from build123d import *

# Parameters (mm, degrees)
EXTRUDE_1_DEPTH         = 5
HOLE_WIZARD_A_0_234_3_D = 3.1999936
PATTERN_LINEAR_1_COUNT  = 3
PATTERN_LINEAR_1_PITCH  = 8
HOLE_WIZARD_A_0_234_4_D = 4


with BuildPart() as part:
    # Эскиз1 → Бобышка-Вытянуть1 (new body)
    with BuildSketch(Plane.XZ):
        with BuildLine():
            Line((-6, 31.613261479), (-6, 0))
            Line((-6, 0), (6, 0))
            Line((6, 0), (6, 37.436574312))
            ThreePointArc((6, 37.436574312), (6.281622528, 39.793084297), (7.110627862, 42.016865021))
            Line((7.110627862, 42.016865021), (12.856242572, 53.167883716))
            ThreePointArc((12.856242572, 53.167883716), (11.13261, 58.555748855), (5.744744861, 56.832116284))
            Line((5.744744861, 56.832116284), (-4.889372139, 36.193552189))
            ThreePointArc((-4.889372139, 36.193552189), (-5.718377472, 33.969771464), (-6, 31.613261479))
        make_face()
    extrude(amount=-EXTRUDE_1_DEPTH)

    # Диаметр отверстия A (0.234)3 (through all)
    with Locations(Plane(origin=(0, 0, 4), x_dir=(0, 0, -1), z_dir=(0, -1, 0))):
        with Locations((0, 0)):
            hole_wizard_a_0_234_3 = Hole(HOLE_WIZARD_A_0_234_3_D / 2)

    # Линейный массив1: Диаметр отверстия A (0.234)3 ×3
    with Locations(*[(0, 0, i * PATTERN_LINEAR_1_PITCH) for i in range(1, PATTERN_LINEAR_1_COUNT)]):
        add(hole_wizard_a_0_234_3, mode=Mode.SUBTRACT)

    # Диаметр отверстия A (0.234)4 (through all)
    with Locations(Plane(origin=(9.3, 0, 55), x_dir=(0, 0, -1), z_dir=(0, -1, 0))):
        with Locations((0, 0), (15.76854256, -8.11912081)):
            Hole(HOLE_WIZARD_A_0_234_4_D / 2)


solid = part.part
Source: CAD feature listing. Evaluate the final solid. Frame: model axes, mm. Coordinates: 2 decimals unless noted, no trailing zeros. Loops run counter-clockwise (first coordinate to the right, second up) from the corner with the lowest first, then second, coordinate; pieces in that order, holes last. Notation, with made-up numbers: (-6.5, 10) -> (52.5, 10) arc R23 ccw to (52.5, 18) -> close; hole circle Ø9 at (68.25, -6.5). An arc over 180 degrees is marked (long way). Answer in a Markdown table with one row per item. Add a question column.
Q1. Section B-B on z = 4. Return the cut outline in (x, y), and give its area (3 significant figures).
Q2. Section C-C on x = 0. Return the cut outline in (y, z), and give its area (3 significant figures).
Q3. Ray query, line 1 along X through (y, z) = (2.2, 4); line 2 along X through (y, z) = (0.3, 6); line 3 along X through (y, z) = (4.6, 55). Return the intervals inside material, ascending.
Q4. Section A-A on x = 10.5. Return the cut outline in (y, z), and give its area (3 significant figures).
Q5. Section D-D on y = 2.05. Return the cut outline in (x, z), and give its area (3 significant figures).
Q6. Pull-direction query (X, two-part tool) for faces 1 (the face through (0, 2, 0)), 2 (the face through (6, 2, 18)), 3 (the face through (0.481, 2.535, 13.526)), 4 (the face through (-6, 2, 16)); classes: pulls with the +X half, pulls with the -X half, needs draft (parallel to the pull), parting line crosses it, or undercut.
Computed values:
| question | item | result |
|---|---|---|
| 1 | outline | (-6, 0) -> (-1.6, 0) -> (-1.6, 5) -> (-6, 5) -> close; (1.6, 0) -> (6, 0) -> (6, 5) -> (1.6, 5) -> close |
| 1 | area | 44.0 mm^2 |
| 2 | outline | (0, 0) -> (5, 0) -> (5, 2.4) -> (0, 2.4) -> close; (0, 5.6) -> (5, 5.6) -> (5, 10.4) -> (0, 10.4) -> close; (0, 13.6) -> (5, 13.6) -> (5, 18.4) -> (0, 18.4) -> close; (0, 21.6) -> (5, 21.6) -> (5, 37.62) -> (0, 37.62) -> close; (0, 40.85) -> (5, 40.85) -> (5, 45.68) -> (0, 45.68) -> close |
| 2 | area | 164 mm^2 |
| 3 | line 1 | x = -6 to -1.6, 1.6 to 6 |
| 3 | line 2 | x = -6 to 6 |
| 3 | line 3 | x = 4.8 to 7.3, 11.3 to 13.3 |
| 4 | outline | (0, 48.59) -> (5, 48.59) -> (5, 53.4) -> (0, 53.4) -> close; (0, 56.6) -> (5, 56.6) -> (5, 58.82) -> (0, 58.82) -> close |
| 4 | area | 35.1 mm^2 |
| 5 | outline | (-6, 0) -> (6, 0) -> (6, 37.44) arc R10 cw to (7.11, 42.02) -> (12.86, 53.17) arc R4 ccw to (5.74, 56.83) -> (-4.89, 36.19) arc R10 ccw to (-6, 31.61) -> close; hole circle Ø3.2 at (0, 4); hole circle Ø3.2 at (0, 12); hole circle Ø3.2 at (0, 20); hole circle Ø4 at (1.18, 39.23); hole circle Ø4 at (9.3, 55) |
| 5 | area | 582 mm^2 |
| 6 | face 1 | needs draft |
| 6 | face 2 | pulls with the +X half |
| 6 | face 3 | undercut |
| 6 | face 4 | pulls with the -X half |
